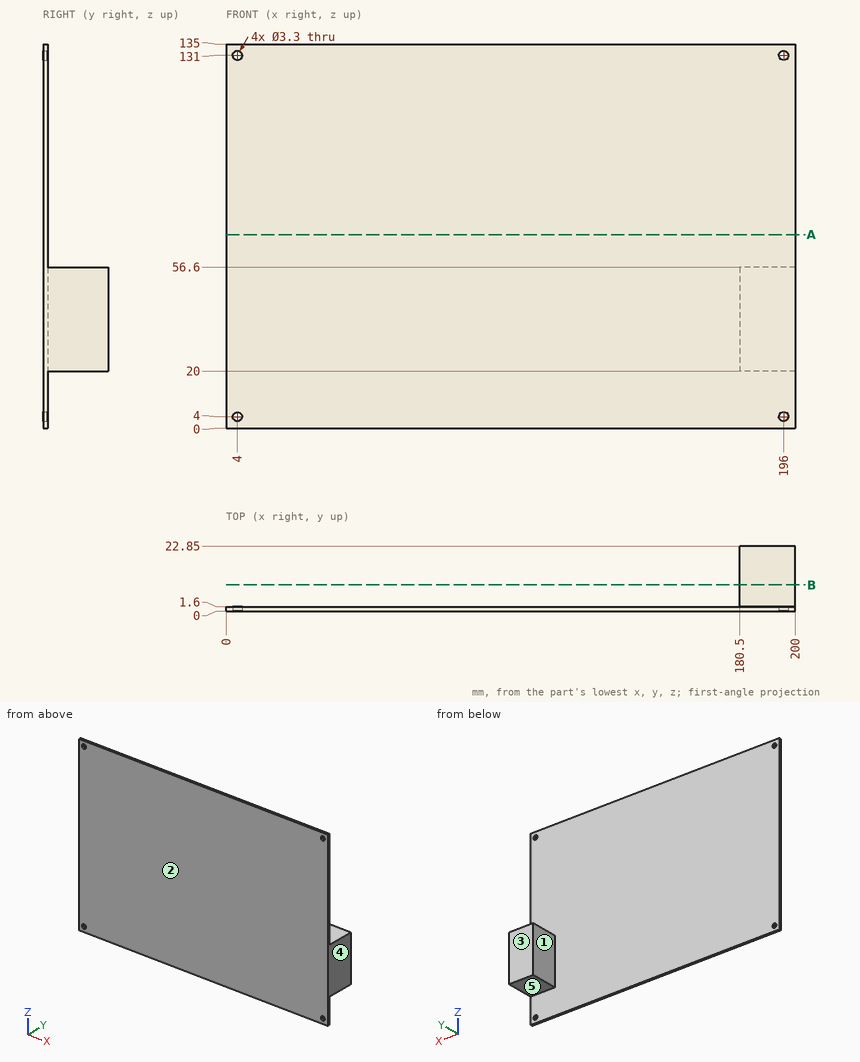
Input: dimensioned drawing with shaded views. Units: mm. Origin: part minimum x, y, z. A direction names the side the tool comes from. Round coordinates to 2 decimals unless told otherwise and drop trailing zeros. Loops run counter-clockwise (first coordinate to the right, second up) from the corner with the lowest first, then second, coordinate; pieces in that order, holes last. Notation, with made-up numbers: M 79,19.5 L 135,19.5 A21 cw 135,52.5 Z; hole C 85.25,27.5 d4. An arc over 180 degrees is marked long. Answer in a Markdown table with one row per item. Add a question column.
1. Section A-A (z = 68). Output: boundary loops of the cut face in (x, y).
2. Section B-B (y = 9.25). Output: boundary loops of the cut face in (x, z).
3. Ray query, probe 1 along X at (y, z) = (0.85, 131); probe 2 along Z at (x, y) = (196, 0.5); probe 3 along Y at (x, z) = (106, 123.5). Return the intervals inside material, ascending.
4. Mould query, pull axis Y, two halves, no side actions, for the marked faces 1, 2 and 3. Classes: released by +Y, released by -Y, zero draft, split by the parting line, or undercut.
5. Set-up query: the marked faces 4 and 5. Return all of +Z, -Z, +X, -X, +Y, -Y with unobstructed straight access to the full face (end or side cutting, diameter ignored); none if empty.
6. Contact query for flat-ended pins moving along their axis: pin 1 (4 mm diameter, centred on x = 196, z = 4, fed in from +Y); pin 2 (10 mm diameter, centred on x = 79, z = 63.5, fed in from -Y); pin 3 (2 mm diameter, centred on y = 9, z = 57.5, fed in from -X); pin 4 (6 mm diameter, centred on x = 187, y = 13, fed in from +Z). Output: stop coordinate, or through.
Values follow:
| question | item | result |
|---|---|---|
| 1 | outline | M 0,0 L 200,0 L 200,1.6 L 0,1.6 Z |
| 2 | outline | M 180.5,20 L 200,20 L 200,56.6 L 180.5,56.6 Z |
| 3 | probe 1 | 0 to 2.35, 5.65 to 194.35, 197.65 to 200 |
| 3 | probe 2 | 0 to 2.35, 5.65 to 129.35, 132.65 to 135 |
| 3 | probe 3 | 0 to 1.6 |
| 4 | face 1 | zero draft |
| 4 | face 2 | released by -Y |
| 4 | face 3 | released by +Y |
| 5 | face 4 | +Z, -Z, +X, +Y, -Y |
| 5 | face 5 | -Z, +X, -X, +Y |
| 6 | pin 1 | y = 1.6 |
| 6 | pin 2 | y = 0 |
| 6 | pin 3 | x = 180.5 |
| 6 | pin 4 | z = 56.6 |
